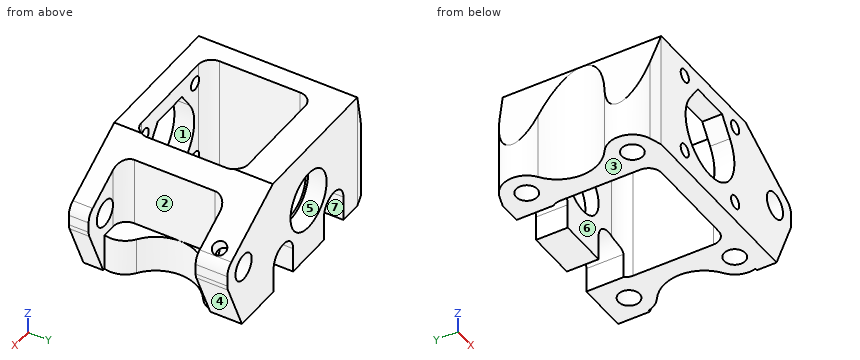
```python
from build123d import *

# Parameters (mm, degrees)
SKETCH1_R           = 9.5
SKETCH1_R_2         = 5
BOSS_EXTRUDE1_DEPTH = 60
SKETCH2_R           = 11.1
CUT_EXTRUDE1_DEPTH  = 7
CUT_EXTRUDE2_DEPTH  = 31
SKETCH4_R           = 2.5
CUT_EXTRUDE3_DEPTH  = 16
SKETCH7_W           = 10.5
SKETCH7_H           = 60
BOSS_EXTRUDE2_DEPTH = 14
BOSS_EXTRUDE3_DEPTH = 60
SKETCH5_R           = 4
CUT_EXTRUDE4_DEPTH  = 13
CUT_EXTRUDE5_DEPTH  = 46.0000001
FILLET1_R           = 5
SKETCH9_R           = 2.6
CUT_EXTRUDE6_DEPTH  = 10
CUT_EXTRUDE7_DEPTH  = 20


with BuildPart() as part:
    # Sketch1 → Boss-Extrude1 (new body)
    with BuildSketch(Plane(origin=(0, 0, 0), x_dir=(1, 0, 0), z_dir=(0, 1, 0))):
        Polygon((-30, 23), (41, 23), (50, 2.057780588), (50, -5.760336739), (22, -22), (-30, -22), align=None)
        with Locations(Location((0, 0, 0), (0, 0, 270))):  # turned: the seam where the file's is
            Circle(SKETCH1_R, mode=Mode.SUBTRACT)
        with Locations(Location((40, 0, 0), (0, 0, 270))):  # turned: the seam where the file's is
            Circle(SKETCH1_R_2, mode=Mode.SUBTRACT)
    extrude(amount=BOSS_EXTRUDE1_DEPTH)

    # Sketch2 → Cut-Extrude1 (cut)
    with BuildSketch(Plane(origin=(0, 60, 0), x_dir=(1, 0, 0), z_dir=(0, 1, 0))):
        with Locations(Location((0, 0, 0), (0, 0, 270))):  # turned: the seam where the file's is
            Circle(SKETCH2_R)
    extrude(amount=-CUT_EXTRUDE1_DEPTH, mode=Mode.SUBTRACT)

    # Sketch3 → Cut-Extrude2 (cut)
    with BuildSketch(Plane.XY.offset(22)):
        with BuildLine():
            Line((-17.5, 48), (17.5, 48))
            ThreePointArc((17.5, 48), (21.035533906, 46.535533906), (22.5, 43))
            Line((22.5, 43), (22.5, 12.5))
            ThreePointArc((22.5, 12.5), (21.035533906, 8.964466094), (17.5, 7.5))
            Line((17.5, 7.5), (-17.5, 7.5))
            ThreePointArc((-17.5, 7.5), (-21.035533906, 8.964466094), (-22.5, 12.5))
            Line((-22.5, 12.5), (-22.5, 43))
            ThreePointArc((-22.5, 43), (-21.035533906, 46.535533906), (-17.5, 48))
        make_face()
        with BuildLine():
            Line((35, 48), (66.370981508, 48))
            Line((66.370981508, 48), (66.370981508, 7.5))
            Line((66.370981508, 7.5), (35, 7.5))
            ThreePointArc((35, 7.5), (31.464466094, 8.964466094), (30, 12.5))
            Line((30, 12.5), (30, 43))
            ThreePointArc((30, 43), (31.464466094, 46.535533906), (35, 48))
        make_face()
    extrude(amount=-CUT_EXTRUDE2_DEPTH, mode=Mode.SUBTRACT)

    # Sketch4 → Cut-Extrude3 (cut)
    with BuildSketch(Plane.XZ):
        with Locations(Location((15.5, 15.5, 0), (0, 0, 270))):  # turned: the seam where the file's is
            Circle(SKETCH4_R)
        with Locations(Location((-15.5, 15.5, 0), (0, 0, 270))):  # turned: the seam where the file's is
            Circle(SKETCH4_R)
        with Locations(Location((-15.5, -15.5, 0), (0, 0, 270))):  # turned: the seam where the file's is
            Circle(SKETCH4_R)
        with Locations(Location((15.5, -15.5, 0), (0, 0, 270))):  # turned: the seam where the file's is
            Circle(SKETCH4_R)
        with BuildLine():
            Line((-12.287280664, 8.603646545), (-7.458401989, 15.5))
            Line((-7.458401989, 15.5), (7.458401989, 15.5))
            Line((7.458401989, 15.5), (12.287280664, 8.603646545))
            ThreePointArc((12.287280664, 8.603646545), (0, -15), (-12.287280664, 8.603646545))
        make_face()
    extrude(amount=-CUT_EXTRUDE3_DEPTH, mode=Mode.SUBTRACT)

    # Sketch7 → Boss-Extrude2 (add)
    with BuildSketch(Plane(origin=(0, 0, -23), x_dir=(-1, 0, 0), z_dir=(0, 0, -1))):
        with Locations((35.25, 30)):
            Rectangle(SKETCH7_W, SKETCH7_H)
    extrude(amount=-BOSS_EXTRUDE2_DEPTH)

    # Sketch8 → Boss-Extrude3 (add)
    with BuildSketch(Plane.XZ):
        Polygon((-40.5, -9), (-30, 22), (-30, -9), align=None)
    extrude(amount=-BOSS_EXTRUDE3_DEPTH)

    # Sketch5 → Cut-Extrude4 (cut)
    with BuildSketch(Plane(origin=(0, 0, -23), x_dir=(-1, 0, 0), z_dir=(0, 0, -1))):
        with Locations((31.5, 50)):
            Circle(SKETCH5_R)
        with Locations((31.5, 10)):
            Circle(SKETCH5_R)
        with Locations((-31.5, 10)):
            Circle(SKETCH5_R)
        with Locations((-31.5, 50)):
            Circle(SKETCH5_R)
    extrude(amount=-CUT_EXTRUDE4_DEPTH, mode=Mode.SUBTRACT)

    # Sketch6 → Cut-Extrude5 (cut, through all)
    with BuildSketch(Plane(origin=(0, 0, -23), x_dir=(-1, 0, 0), z_dir=(0, 0, -1))):
        with BuildLine():
            Line((17.5, 48), (-17.5, 48))
            ThreePointArc((-17.5, 48), (-21.035533906, 46.535533906), (-22.5, 43))
            Line((-22.5, 43), (-22.5, 12.5))
            ThreePointArc((-22.5, 12.5), (-21.035533906, 8.964466094), (-17.5, 7.5))
            Line((-17.5, 7.5), (17.5, 7.5))
            ThreePointArc((17.5, 7.5), (21.035533906, 8.964466094), (22.5, 12.5))
            Line((22.5, 12.5), (22.5, 43))
            ThreePointArc((22.5, 43), (21.035533906, 46.535533906), (17.5, 48))
        make_face()
        with BuildLine():
            Line((34.369237169, 58.530385575), (30, 60))
            Line((30, 60), (30, 65.619685256))
            Line((30, 65.619685256), (48.74877155, 65.619685256))
            Line((48.74877155, 65.619685256), (48.74877155, -4.23456535))
            Line((48.74877155, -4.23456535), (30, -4.23456535))
            Line((30, -4.23456535), (30, 0))
            Line((30, 0), (34.369237169, 1.469614425))
            ThreePointArc((34.369237169, 1.469614425), (40.412298518, 8.746630491), (36.610730034, 17.408133268))
            ThreePointArc((36.610730034, 17.408133268), (30, 30), (36.610730034, 42.591866732))
            ThreePointArc((36.610730034, 42.591866732), (40.412298518, 51.253369509), (34.369237169, 58.530385575))
        make_face()
        with BuildLine():
            Line((-50, 48), (-40.274964387, 48))
            ThreePointArc((-40.274964387, 48), (-38.950845842, 44.951743247), (-36.610730034, 42.591866732))
            ThreePointArc((-36.610730034, 42.591866732), (-30, 30), (-36.610730034, 17.408133268))
            ThreePointArc((-36.610730034, 17.408133268), (-39.976636272, 13.024340839), (-40.145808233, 7.5))
            Line((-40.145808233, 7.5), (-50, 7.5))
            Line((-50, 7.5), (-50, 48))
        make_face()
    extrude(amount=-CUT_EXTRUDE5_DEPTH, mode=Mode.SUBTRACT)

    # Fillet1
    fillet1_edges = [part.edges().sort_by_distance(p)[0] for p in [
        (50, 54, -2.057780588),
        (50, 54, 5.760336739),
        (50, 3.75, -2.057780588),
        (50, 3.75, 5.760336739),
    ]]
    fillet(fillet1_edges, radius=FILLET1_R)

    # Sketch9 → Cut-Extrude6 (cut)
    with BuildSketch(Plane(origin=(15.085632266, 0, 26.010250131), x_dir=(0.865035704, 0, -0.501710305), z_dir=(0.501710305, 0, 0.865035704))):
        with Locations((34.60142817, 54)):
            Circle(SKETCH9_R)
    extrude(amount=-CUT_EXTRUDE6_DEPTH, mode=Mode.SUBTRACT)

    # Sketch10 → Cut-Extrude7 (cut)
    with BuildSketch(Plane(origin=(0, 60, 0), x_dir=(1, 0, 0), z_dir=(0, 1, 0))):
        with BuildLine():
            Line((21.5, 23), (9.5, 23))
            Line((9.5, 23), (9.5, 13.5))
            ThreePointArc((9.5, 13.5), (15.5, 7.5), (21.5, 13.5))
            Line((21.5, 13.5), (21.5, 23))
        make_face()
        with BuildLine():
            Line((-21.5, 13.5), (-21.5, 23))
            Line((-21.5, 23), (-9.5, 23))
            Line((-9.5, 23), (-9.5, 13.5))
            ThreePointArc((-9.5, 13.5), (-15.5, 7.5), (-21.5, 13.5))
        make_face()
    extrude(amount=-CUT_EXTRUDE7_DEPTH, mode=Mode.SUBTRACT)


solid = part.part
```
The listing builds one solid part. Answer for the finished solid, in the listing's coordinates (mm). Face numbers are marked on the shaded views. A direction names the side the tool comes from. Give positions to 0.01 mm unless a question says otherwise; leave off trailing zeros. Loops run counter-clockwise (first coordinate to the right, second up) from the corner with the lowest first, then second, coordinate; pieces in that order, holes last. Notation, with made-up numbers: (55, 46.5) - (76, 46.5) arc R18 cw to (76, 81.5) - close; hole circle Ø3 at (27.5, -33). An arc over 180 degrees is marked (long way). Return JSON: item names as keys, results as strings. Group by question number.
1. Find section C-C (z = 19.5). Write down the section's boundary in (x, y).
2. Given pin 1 Ø3 at (y, z) = (52, -19) entering from -X; pin 2 Ø9 at (x, y) = (31.5, 10) entering from -Z; pin 3 Ø5 at (y, z) = (49.5, -17.5) entering from +X; pin 4 Ø10 at (y, z) = (16, 8.5) entering from -X, each flat-ended and moving along its own axis, determine where each tip first touches the part or whether it passes through.
3. Which of the six approach directions +Z, -Z, +X, -X, +Y, -Y give full straight-line access (tool end or side, diameter ignored) to the marked faces 4, 5, 6 and 7?
4. Determine the mould class of the marked faces 1, 2 and 3 for opening direction X: pulls with the +X half, pulls with the -X half, needs draft (parallel to the pull), parting line crosses it, or undercut.
5. Find section A-A (y = 50). Write down the section's boundary in (x, z), then the cut area to 3 significant figures.
6. Straight lines are drawn through the part: line 1 (Z direction, x = -15.5, y = 3.75); line 2 (X direction, y = 57.5, z = 0); line 3 (X direction, y = 5.25, z = -15.5). For each, find the intervals that lie inside material, in ascending order. Write a range as [from, to].
7. Find section B-B (x = 31.5). Write down the section's boundary in (y, z), then the cut area to 3 significant figures.
8. Find section D-D (y = 21.5). Write down the section's boundary in (x, z), then the cut area to 3 significant figures.
Verdict:
{
 "1": {"outline": "(-30.85, 0.28) - (-30, 0) - (26.31, 0) - (26.31, 60) - (-30, 60) - (-30.85, 59.72) - (-30.85, 35.02) arc R15.3 cw to (-30.85, 24.98) - close; hole (-22.5, 12.5) arc R5 ccw to (-17.5, 7.5) - (17.5, 7.5) arc R5 ccw to (22.5, 12.5) - (22.5, 43) arc R5 ccw to (17.5, 48) - (-17.5, 48) arc R5 ccw to (-22.5, 43) - close"},
 "2": {"pin 1": "stops at x = -40.49", "pin 2": "stops at z = -23", "pin 3": "stops at x = 44.44", "pin 4": "stops at x = -36.27"},
 "3": {"face 4": "-Z, +X, +Y, -Y", "face 5": "+Y", "face 6": "+Z, -Z", "face 7": "-Z, +Y"},
 "4": {"face 1": "undercut", "face 2": "pulls with the +X half", "face 3": "needs draft"},
 "5": {"outline": "(-40.5, -23) - (-35.5, -23) - (-35.5, -10) - (-27.5, -10) - (-27.5, -23) - (-21.5, -23) - (-21.5, -13.5) arc R6 cw to (-9.5, -13.5) - (-9.5, -23) - (9.5, -23) - (9.5, -13.5) arc R6 cw to (21.5, -13.5) - (21.5, -23) - (27.5, -23) - (27.5, -10) - (35.5, -10) - (35.5, -23) - (41, -23) - (49.59, -3) arc R5 ccw to (50, -1.03) - (50, 2.88) arc R5 ccw to (47.51, 7.21) - (22, 22) - (-30, 22) - (-40.5, -9) - close; hole circle Ø19 at (0, 0); hole circle Ø10 at (40, 0)", "area": "2,680 mm^2"},
 "6": {"line 1": "z = [-23, -18], [-13, 13], [18, 22]", "line 2": "x = [-36.47, -11.1], [11.1, 35], [45, 50]", "line 3": "x = [-39.14, -18], [-13, 13], [18, 44.22]"},
 "7": {"outline": "(0, -23) - (6, -23) - (6, -10) - (14, -10) - (14, -23) - (23.39, -23) - (23.39, -9) - (8.93, -9) - (8.93, 16.49) - (0, 16.49) - close; (36.61, -23) - (46, -23) - (46, -10) - (54, -10) - (54, -23) - (60, -23) - (60, 16.49) - (46.57, 16.49) - (46.57, -9) - (36.61, -9) - close", "area": "1,020 mm^2"},
 "8": {"outline": "(-32.58, -23) - (-22.5, -23) - (-22.5, 22) - (-30, 22) - (-32.58, 14.39) - close; (22.5, -23) - (32.58, -23) - (32.58, -9) - (30, -9) - (30, 17.36) - (22.5, 21.71) - close", "area": "799 mm^2"}
}
